from build123d import *

# Parameters (mm, degrees)
SKETCH_1_R               = 7.5
EXTRUDE_1_DEPTH          = 0.5
SKETCH_2_R               = 6.115
EXTRUDE_2_DEPTH          = 7
CUT_EXTRUDE_3_DEPTH      = 7
SKETCH_3_R               = 7.5
EXTRUDE_3_DEPTH          = 1
SKETCH_6_R               = 2.5
CUT_EXTRUDE_2_DEPTH      = 10
PATTERN_CIRCULAR_2_COUNT = 20


with BuildPart() as part:
    # 草圖1 → 填料-伸長1 (new body, symmetric)
    with BuildSketch(Plane.XY):
        Circle(SKETCH_1_R)
    extrude(amount=EXTRUDE_1_DEPTH, both=True)

    # 草圖2 → 填料-伸長2 (add)
    with BuildSketch(Plane.XY.offset(0.5)):
        Circle(SKETCH_2_R)
    extrude(amount=EXTRUDE_2_DEPTH)

    # 草圖7 → 除料-伸長3 (cut)
    with BuildSketch(Plane.XY.offset(7.5)):
        with BuildLine():
            ThreePointArc((-0.599277509, 6.085564186), (0, 5.515), (0.599277509, 6.085564186))
            ThreePointArc((0.599277509, 6.085564186), (0, 6.115), (-0.599277509, 6.085564186))
        make_face()
    cut_extrude_3 = extrude(amount=-CUT_EXTRUDE_3_DEPTH, mode=Mode.SUBTRACT)

    # 草圖3 → 填料-伸長3 (add)
    with BuildSketch(Plane.XY.offset(7.5)):
        Circle(SKETCH_3_R)
    extrude(amount=EXTRUDE_3_DEPTH)

    # 草圖6 → 除料-伸長2 (cut, through all)
    with BuildSketch(Plane(origin=(0, 0, -0.5), x_dir=(-1, 0, 0), z_dir=(0, 0, -1))):
        Circle(SKETCH_6_R)
    extrude(amount=-CUT_EXTRUDE_2_DEPTH, mode=Mode.SUBTRACT)

    # 環狀複製排列2: 除料-伸長3 ×20 about axis
    pattern_circular_2_axis = Axis((0, 0, 0), (0, 0, 1))
    for i in range(1, PATTERN_CIRCULAR_2_COUNT):
        add(cut_extrude_3.rotate(pattern_circular_2_axis, i * 360 / PATTERN_CIRCULAR_2_COUNT), mode=Mode.SUBTRACT)


solid = part.part
Verification items for the finished model (mm, model axes). A direction names the side the tool comes from. Give positions to 0.01 mm unless a question says otherwise; leave off trailing zeros. Write each loop counter-clockwise with the first axis right and the second up, starting at its lowest first coordinate (ties: lowest second). Pieces come first, ordered by that corner, then holes. Notation, with made-up numbers: M 13,-16 L 26,-16 A17 cw 26,2 Z; hole C 30,64 d9. An arc over 180 degrees is marked long. Use CSV: the item, a comma, the result in double quotes.
1) Go/stop test with flat-tipped pins: pin 1 Ø2 at (x, z) = (-0.5, 7.5) entering from +Y; pin 2 Ø1 at (x, z) = (-2.5, 5.5) entering from +Y. Record where each tip stops, or that it passes through.
Final values:
pin 1,"y = 7.5"
pin 2,"y = 5.6"
2) Material ranges on line 1 along Z through (x, y) = (1.5, 6.5); line 2 along Y through (x, z) = (0, 3) (3 decimals); line 3 along X through (y, z) = (1.5, 6.5), recorded low to high.
Final values:
line 1,"-0.5 to 0.5, 7.5 to 8.5"
line 2,"-5.515 to -2.5, 2.5 to 5.515"
line 3,"-5.36 to -2, 2 to 5.36"
3) Release check for a two-part mould opening along Y. For faces 1 (the face through (-7.493, 0.33, 0.007)), 2 (the face through (-2, 2, 8.5)), 3 (the face through (-5.25, 1.69, 4.05)) record: released by +Y, released by -Y, zero draft, split by the parting line, or undercut.
Final values:
face 1,"split by the parting line"
face 2,"zero draft"
face 3,"undercut"
4) Cross-section at C-C (x = 3.75). Enter the section's corners in (y, z), plus the area to 3 significant figures.
Final values:
outline,"M -6.5,-0.5 L 6.5,-0.5 L 6.5,0.5 L 4.37,0.5 L 4.37,7.5 L 6.5,7.5 L 6.5,8.5 L -6.5,8.5 L -6.5,7.5 L -4.37,7.5 L -4.37,0.5 L -6.5,0.5 Z"
area,"87.1 mm²"
5) Cross-section at A-A (x = 0). Enter the section's corners in (y, z) (3 decimals).
Final values:
outline,"M -7.5,-0.5 L -2.5,-0.5 L -2.5,8.5 L -7.5,8.5 L -7.5,7.5 L -5.515,7.5 L -5.515,0.5 L -7.5,0.5 Z; M 2.5,-0.5 L 7.5,-0.5 L 7.5,0.5 L 5.515,0.5 L 5.515,7.5 L 7.5,7.5 L 7.5,8.5 L 2.5,8.5 Z"
6) Access from +Z, -Z, +X, -X, +Y, -Y to the whole of each face (thin tool, end or side, straight path). Record for faces 4 (the face through (5.515, 0.013, 4.049)), 5 (the face through (0.54, -2.44, 3.94)), 6 (the face through (4.454, 3.252, 4.049)).
Final values:
face 4,"+X"
face 5,"+Z, -Z"
face 6,"none"
